The listing builds one solid part. Answer for the finished solid, in the listing's coordinates (mm). A direction names the side the tool comes from. Give positions to 0.01 mm unless a question says otherwise; leave off trailing zeros. Write each loop counter-clockwise with the first axis right and the second up, starting at its lowest first coordinate (ties: lowest second). Pieces come first, ordered by that corner, then holes.
```python
from build123d import *

# Parameters (mm, degrees)
F0_R     = 5
F1_DEPTH = 30
F2_DEPTH = 40


with BuildPart() as f1:
    # F0 (on Front) → F1 (new body)
    with BuildSketch(Plane.XZ):
        with BuildLine():
            Line((-40, 25), (-25.980762, 25))
            ThreePointArc((-25.980762, 25), (-28.977775, 32.235429), (-30, 40))
            Line((-30, 40), (-40, 40))
            Line((-40, 40), (-40, 25))
        make_face()
        with BuildLine():
            ThreePointArc((30, 40), (21.213203, 18.786797), (0, 10))
            Line((0, 10), (0, 0))
            Line((0, 0), (40, 0))
            Line((40, 0), (40, 40))
            Line((40, 40), (30, 40))
        make_face()
        with Locations((30, 10)):
            Circle(F0_R, mode=Mode.SUBTRACT)
    extrude(amount=F1_DEPTH)

    # F0 (on Front) → F2 (join)
    with BuildSketch(Plane.XZ):
        with BuildLine():
            Line((0, 0), (0, 10))
            ThreePointArc((0, 10), (-15, 14.019238), (-25.980762, 25))
            Line((-25.980762, 25), (-40, 25))
            Line((-40, 25), (-40, 0))
            Line((-40, 0), (0, 0))
        make_face()
        with Locations((-30, 10)):
            Circle(F0_R, mode=Mode.SUBTRACT)
    extrude(amount=F2_DEPTH)


solid = f1.part
```
Item 1: Determine the mould class of faces 4 (the face through (0, -35, 5)), 5 (the face through (-35, -15, 40)), 6 (the face through (25, -15, 10)) for opening direction X: pulls with the +X half, pulls with the -X half, needs draft (parallel to the pull), parting line crosses it, or undercut.
Conclusion:
face 4: pulls with the +X half
face 5: needs draft
face 6: undercut
Item 2: A cutting plane is placed at D-D, the plane z = 24. Give the vertices of the cut face in (x, y), plus the area to 3 significant figures.
Conclusion:
outline: (-40, -40) - (-25.38, -40) - (-25.38, 0) - (-40, 0) - close; (25.38, -30) - (40, -30) - (40, 0) - (25.38, 0) - close
area: 1,020 mm2
Item 3: Consider probe 1 along X at (y, z) = (-25, 14); probe 2 along X at (y, z) = (-16, 8); probe 3 along Y at (x, z) = (29, 2). Determine where each line is inside the solid, lowest interval first.
Conclusion:
probe 1: x = -40 to -33, -27 to -14.97, 14.97 to 27, 33 to 40
probe 2: x = -40 to -34.58, -25.42 to 25.42, 34.58 to 40
probe 3: y = -30 to 0
Item 4: Each of these flat-tipped pins is pushed along its axis until it touches: P1, Ø12, axis at x = 28, z = 19, coming from the -Y side; P2, Ø3, axis at x = -33, y = -36.5, coming from the +Z side; P3, Ø11, axis at y = -36, z = 7, coming from the +X side; P4, Ø8, axis at x = -30, z = 10, coming from the -Y side. Where does it stop, or does it pass through?
Conclusion:
P1: stops at y = -30
P2: stops at z = 25
P3: stops at x = 0
P4: passes through
Item 5: A cutting plane is placed at C-C, the plane x = -27. Give the vertices of the cut face in (y, z), plus the area to 3 significant figures.
Conclusion:
outline: (-40, 0) - (0, 0) - (0, 6) - (-40, 6) - close; (-40, 14) - (0, 14) - (0, 26.92) - (-30, 26.92) - (-30, 25) - (-40, 25) - close
area: 738 mm2
Item 6: A cutting plane is placed at A-A, the plane z = 7. Give the vertices of the cut face in (x, y), plus the area to 3 significant figures.
Conclusion:
outline: (-40, -40) - (-34, -40) - (-34, 0) - (-40, 0) - close; (-26, -40) - (0, -40) - (0, -30) - (26, -30) - (26, 0) - (-26, 0) - close; (34, -30) - (40, -30) - (40, 0) - (34, 0) - close
area: 2,240 mm2
Item 7: Which of the six approach directions +Z, -Z, +X, -X, +Y, -Y give full straight-line access (tool end or side, diameter ignored) to faces 1 (the face through (-40, -20, 20)), 2 (the face through (-33, -35, 25)), 3 (the face through (24, -30, 16))?
Conclusion:
face 1: +Z, -Z, -X, +Y, -Y
face 2: +Z, +X, -X, -Y
face 3: +Z, -Z, +X, -Y
Item 8: A cutting plane is placed at B-B, the plane y = -26.5. Give the vertices of the cut face in (x, z), plus the area to 3 significant figures.
Conclusion:
outline: (-40, 0) - (40, 0) - (40, 40) - (30, 40) arc R30 cw to (0, 10) arc R30 cw to (-25.98, 25) arc R30 cw to (-30, 40) - (-40, 40) - close; hole circle Ø10 at (-30, 10); hole circle Ø10 at (30, 10)
area: 1,630 mm2
